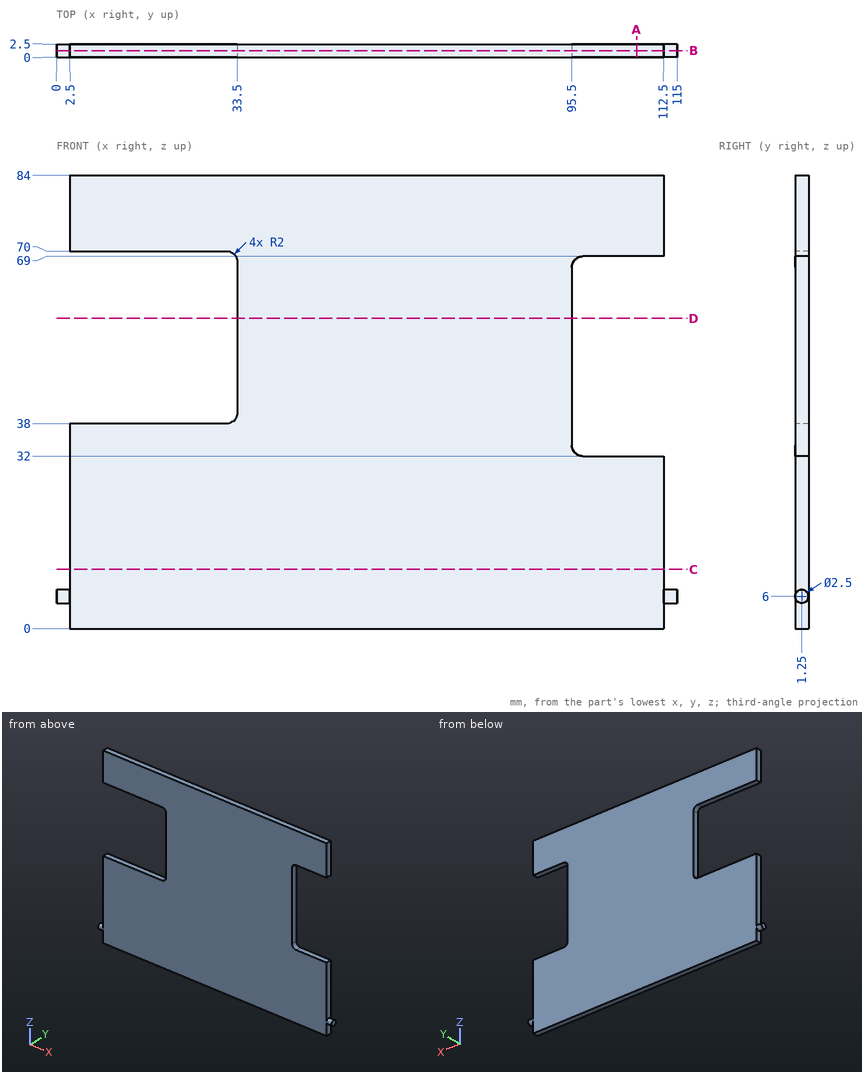
Here's the drawing with two shaded views (mm, measured from the low corner). I have some questions. Coordinates: 2 decimals unless noted, no trailing zeros. Write each loop counter-clockwise with the first axis right and the second up, starting at its lowest first coordinate (ties: lowest second). Pieces come first, ordered by that corner, then holes. Notation, with made-up numbers: (-27, -33.75) - (-14, -33.75) arc R34 ccw to (-14, 2.25) - close; hole circle Ø10 at (79, -33.5). An arc over 180 degrees is marked (long way). Return JSON: item names as keys, results as strings.
Q1. If we section it at A-A (x = 107.5): Please give me the cut outline in (y, z).
Computed values:
{"outline": "(0, 0) - (2.5, 0) - (2.5, 32) - (0, 32) - close; (0, 69) - (2.5, 69) - (2.5, 84) - (0, 84) - close"}
Q2. I'm going to push flat-ended pins straight in: pin 1 Ø1.2 at (y, z) = (1.5, 2.5) entering from -X; pin 2 Ø0.8 at (y, z) = (1, 52.5) entering from -X; pin 3 Ø1.2 at (y, z) = (1, 3) entering from +X. Where does each tip first touch, or does it pass through?
Computed values:
{"pin 1": "stops at x = 2.5", "pin 2": "stops at x = 33.5", "pin 3": "stops at x = 112.5"}
Q3. Please list where these lines run through material, in increasing order: L1, parallel to Z at x = 10.5, y = 2; L2, parallel to X at y = 1, z = 21.5; L3, parallel to X at y = 1.15, z = 36. Write a range as from..to.
Computed values:
{"L1": "z = 0..38, 70..84", "L2": "x = 2.5..112.5", "L3": "x = 2.5..95.5"}
Q4. If we section it at C-C (z = 11): Please give me the cut outline in (x, y), then the cut area to 3 significant figures.
Computed values:
{"outline": "(2.5, 0) - (112.5, 0) - (112.5, 2.5) - (2.5, 2.5) - close", "area": "275 mm2"}
Q5. If we section it at B-B (y = 1.25): Please give me the cut outline in (x, z).
Computed values:
{"outline": "(0, 4.75) - (2.5, 4.75) - (2.5, 0) - (112.5, 0) - (112.5, 4.75) - (115, 4.75) - (115, 7.25) - (112.5, 7.25) - (112.5, 32) - (97.5, 32) arc R2 cw to (95.5, 34) - (95.5, 67) arc R2 cw to (97.5, 69) - (112.5, 69) - (112.5, 84) - (2.5, 84) - (2.5, 70) - (31.5, 70) arc R2 cw to (33.5, 68) - (33.5, 40) arc R2 cw to (31.5, 38) - (2.5, 38) - (2.5, 7.25) - (0, 7.25) - close"}
Q6. If we section it at D-D (z = 57.5): Please give me the cut outline in (x, y).
Computed values:
{"outline": "(33.5, 0) - (95.5, 0) - (95.5, 2.5) - (33.5, 2.5) - close"}
